Could you check a few things on this model? Use its own coordinates, in mm. Face numbers are marked on the shaded views. A direction names the side the tool comes from. Give positions to 0.01 mm unless a question says otherwise; leave off trailing zeros. Loops run counter-clockwise (first coordinate to the right, second up) from the corner with the lowest first, then second, coordinate; pieces in that order, holes last. Notation, with made-up numbers: M -14.75,15 L 6.25,15 A34 cw 6.25,54 Z; hole C -26,-31.75 d2. An arc over 180 degrees is marked long. Use CSV: the item, a comma, the result in double quotes.
```python
from build123d import *

# Parameters (mm, degrees)
SKETCH1_R               = 3.1623
BOSS_EXTRUDE1_DEPTH     = 11.0998
CUT_EXTRUDE1_DEPTH      = 1
CUT_EXTRUDE1_DEPTH_BACK = 12.0998
SKETCH3_R               = 6.35
BOSS_EXTRUDE2_DEPTH     = 73.279


with BuildPart() as part:
    # Sketch1 → Boss-Extrude1 (new body)
    with BuildSketch(Plane.XY):
        Circle(SKETCH1_R)
    extrude(amount=BOSS_EXTRUDE1_DEPTH)

    # Sketch2 → Cut-Extrude1 (cut, two sides)
    with BuildSketch(Plane(origin=(0, 0, 0), x_dir=(-1, 0, 0), z_dir=(0, 0, -1))) as cut_extrude1_sk:
        Polygon((17.073178183, -20.234228338), (0.001249598, -3.162299753), (-3.162299753, 0.001249598), (-20.234228338, 17.073178183), (-54.378085507, -17.070678986), (-17.070678986, -54.378085507), align=None)
    extrude(amount=CUT_EXTRUDE1_DEPTH, mode=Mode.SUBTRACT)
    extrude(cut_extrude1_sk.sketch, amount=-CUT_EXTRUDE1_DEPTH_BACK, mode=Mode.SUBTRACT)

    # Sketch3 → Boss-Extrude2 (add)
    with BuildSketch(Plane.XY.offset(11.0998)):
        Circle(SKETCH3_R)
    extrude(amount=BOSS_EXTRUDE2_DEPTH)


solid = part.part
```
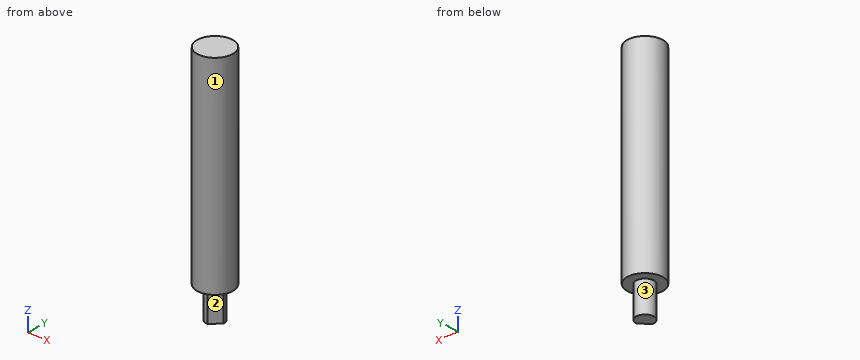
1. I want a section at A-A, the plane y = 1.25. List the corners of the cut face in (x, z) for me, then the cut area to 3 significant figures.
Outcome:
outline,"M -6.23,11.1 L -2.9,11.1 L -2.9,0 L 2.9,0 L 2.9,11.1 L 6.23,11.1 L 6.23,84.38 L -6.23,84.38 Z"
area,"977 mm2"
2. I want a section at D-D, the plane x = -5. List the corners of the cut face in (y, z) for me.
Outcome:
outline,"M -3.91,11.1 L 3.91,11.1 L 3.91,84.38 L -3.91,84.38 Z"
3. I want a section at B-B, the plane x = -1.5. List the corners of the cut face in (y, z) for me.
Outcome:
outline,"M -6.17,11.1 L -2.78,11.1 L -2.78,0 L 2.78,0 L 2.78,11.1 L 6.17,11.1 L 6.17,84.38 L -6.17,84.38 Z"
4. Which directions (+Z, -Z, +X, -X, +Y, -Y) give clear straight access to the entire face, cutting with the end or side of a thin tool? Please do the marked faces 1, 2 and 3.
Outcome:
face 1,"+Z, -Z"
face 2,"-Z, +X, -Y"
face 3,"-Z"
5. I want a section at C-C, the plane z = 52.5. List the corners of the cut face in (x, y) for me.
Outcome:
outline,"C 0,0 d12.7"
6. I'm going to push flat-ended pins straight in: pin 1 Ø4 at (x, y) = (0, 1) entering from -Z; pin 2 Ø5 at (x, z) = (4, 50.5) entering from +Y; pin 3 Ø1 at (x, y) = (1.5, -3.5) entering from -Z; pin 4 Ø1.5 at (y, z) = (2, 31.5) entering from -X. Where does each tip first touch, or does it pass through?
Outcome:
pin 1,"z = 0"
pin 2,"y = 6.17"
pin 3,"z = 11.1"
pin 4,"x = -6.23"
7. Please list where these lines run through material, in increasing order: line 1 (Z direction, x = 4.25, y = -2); line 2 (X direction, y = -0.25, z = 14.5); line 3 (X direction, y = -5.5, z = 23).
Outcome:
line 1,"11.1 to 84.38"
line 2,"-6.35 to 6.35"
line 3,"-3.17 to 3.17"
